```python
from build123d import *

# Parameters (mm, degrees)
SKETCH_1_W                = 50.28
SKETCH_1_H                = 34.2
SKETCH_1_W_2              = 30.28
SKETCH_1_H_2              = 14.2
EXTRUDE_1_DEPTH           = 12.25
SKETCH_4_W                = 13
SKETCH_4_H                = 13.91
EXTRUDE_1_2_DEPTH         = 74.82
SKETCH_5_W                = 13.91
SKETCH_5_H                = 16.23
EXTRUDE_2_DEPTH           = 16
SKETCH_7_R                = 25.25
SKETCH_7_R_2              = 15.25
EXTRUDE_2_2_DEPTH         = 16.23
SKETCH_15_R               = 1.91
CUT_EXTRUDE_6_DEPTH       = 97.964478439
SKETCH_18_W               = 49.344544624
SKETCH_18_H               = 6.125
CUT_EXTRUDE_8_DEPTH       = 101.789238284
SKETCH_19_W               = 34.2
SKETCH_19_H               = 6.125
CUT_EXTRUDE_9_DEPTH       = 10
SKETCH_21_R               = 1.91
CUT_EXTRUDE_10_DEPTH      = 10
SKETCH_20_R               = 1.91
CUT_EXTRUDE_11_DEPTH      = 10
FILLET_START              = -7.1
FILLET_1_DEPTH            = 14.2
FILLET_2_DEPTH            = 14.2
SKETCH_29_W               = 13.91
SKETCH_29_H               = 74.82
EXTRUDE_5_DEPTH           = 10
SKETCH_30_W               = 10
SKETCH_30_H               = 58.59
CUT_EXTRUDE_13_DEPTH      = 97.964478439
SKETCH_32_W               = 34.2
SKETCH_32_H               = 5.745736365
EXTRUDE_6_DEPTH           = 10
CUT_EXTRUDE_16_DEPTH      = 50
CUT_EXTRUDE_16_DEPTH_BACK = 50
SKETCH_38_W               = 116.985630298
SKETCH_38_H               = 80.538350638
SKETCH_41_W               = 13.91
SKETCH_41_H               = 5.745736365
EXTRUDE_7_DEPTH           = 3
SKETCH_42_W               = 13
SKETCH_42_H               = 13.91
EXTRUDE_8_DEPTH           = 74.82
SKETCH_43_W               = 13.91
SKETCH_43_H               = 16.23
EXTRUDE_9_DEPTH           = 15.22
SKETCH_44_R               = 1.91
CUT_EXTRUDE_17_DEPTH      = 15.22
SKETCH_46_R               = 25.25
SKETCH_46_R_2             = 15.25
EXTRUDE_6_2_DEPTH         = 16.23
EXTRUDE_10_DEPTH          = 7.22
EXTRUDE_10_DEPTH_BACK     = 10
SKETCH_47_W               = 13.91
SKETCH_47_H               = 16.23
SKETCH_50_W               = 3.056753925
SKETCH_50_H               = 16.23
CUT_EXTRUDE_18_DEPTH      = 96.578211037
SKETCH_51_R               = 1.91
CUT_EXTRUDE_19_DEPTH      = 95.015226304
SKETCH_52_W               = 92.841945613
SKETCH_52_H               = 30
CUT_EXTRUDE_20_DEPTH      = 84.840694713
CUT_EXTRUDE_22_DEPTH      = 50
CUT_EXTRUDE_22_DEPTH_BACK = 50
SKETCH_53_W               = 63.541345486
SKETCH_53_H               = 14.170740414
SKETCH_54_W               = 10
SKETCH_54_H               = 10.145
CUT_EXTRUDE_23_DEPTH      = 50
SKETCH_55_W               = 13
SKETCH_55_H               = 13.91
EXTRUDE_11_DEPTH          = 10
SKETCH_57_W               = 15
SKETCH_57_H               = 34.2
EXTRUDE_12_DEPTH          = 10
SKETCH_58_W               = 34.2
SKETCH_58_H               = 10
EXTRUDE_13_DEPTH          = 27.85
SKETCH_60_W               = 34.2
SKETCH_60_H               = 10
EXTRUDE_14_DEPTH          = 50.28
SKETCH_62_W               = 30.28
SKETCH_62_H               = 14.2
CUT_EXTRUDE_24_DEPTH      = 50.28
SKETCH_64_R               = 1.91
CUT_EXTRUDE_25_DEPTH      = 10
FILLET_3_R                = 30


with BuildPart() as part:
    # 草圖1 → Extrude 1 (new body)
    with BuildSketch(Plane(origin=(0, 0, 0), x_dir=(1, 0, 0), z_dir=(0, 1, 0))):
        Rectangle(SKETCH_1_W, SKETCH_1_H)
        Rectangle(SKETCH_1_W_2, SKETCH_1_H_2, mode=Mode.SUBTRACT)
    extrude(amount=EXTRUDE_1_DEPTH)

    # 草圖4 → Extrude 1 2 (add)
    with BuildSketch(Plane.XZ):
        with Locations((18.64, 0)):
            Rectangle(SKETCH_4_W, SKETCH_4_H)
    extrude(amount=EXTRUDE_1_2_DEPTH)

    # 草圖5 → Extrude 2 (add)
    with BuildSketch(Plane.ZY.offset(-12.14)):
        with Locations((0, -66.705)):
            Rectangle(SKETCH_5_W, SKETCH_5_H)
    extrude(amount=EXTRUDE_2_DEPTH)

    # 草圖7 → Extrude 2 2 (add)
    with BuildSketch(Plane(origin=(3.626674765, -74.82, 0), x_dir=(1, 0, 0), z_dir=(0, -1, 0))):
        with Locations((-30.978154344, 0)):
            Circle(SKETCH_7_R)
        with Locations((-30.978154344, 0)):
            Circle(SKETCH_7_R_2, mode=Mode.SUBTRACT)
    extrude(amount=-EXTRUDE_2_2_DEPTH)

    # 草圖15 → 除料-伸長6 (cut, through all)
    with BuildSketch(Plane(origin=(0, 0, -6.955), x_dir=(-1, 0, 0), z_dir=(0, 0, -1))):
        with Locations((-4.530883248, -66.705)):
            Circle(SKETCH_15_R)
    extrude(amount=-CUT_EXTRUDE_6_DEPTH, mode=Mode.SUBTRACT)

    # 草圖18 → 除料-伸長8 (cut, through all)
    with BuildSketch(Plane(origin=(0, 0, -17.1), x_dir=(-1, 0, 0), z_dir=(0, 0, -1))):
        with Locations((0.467727688, 9.1875)):
            Rectangle(SKETCH_18_W, SKETCH_18_H)
    extrude(amount=-CUT_EXTRUDE_8_DEPTH, mode=Mode.SUBTRACT)

    # 草圖19 → 除料-伸長9 (cut)
    with BuildSketch(Plane.ZY.offset(-24.204544624)):
        with Locations((0, 9.1875)):
            Rectangle(SKETCH_19_W, SKETCH_19_H)
    extrude(amount=-CUT_EXTRUDE_9_DEPTH, mode=Mode.SUBTRACT)

    # 草圖21 → 除料-伸長10 (cut)
    with BuildSketch(Plane(origin=(0, 6.125, 0), x_dir=(1, 0, 0), z_dir=(0, 1, 0))):
        with Locations(Location((17.69, 0, 0), (0, 0, 270))):
            Circle(SKETCH_21_R)
    extrude(amount=-CUT_EXTRUDE_10_DEPTH, mode=Mode.SUBTRACT)

    # 草圖20 → 除料-伸長11 (cut)
    with BuildSketch(Plane(origin=(0, 6.125, 0), x_dir=(1, 0, 0), z_dir=(0, 1, 0))):
        with Locations(Location((-17.395, 0, 0), (0, 0, 270))):
            Circle(SKETCH_20_R)
    extrude(amount=-CUT_EXTRUDE_11_DEPTH, mode=Mode.SUBTRACT)

    # 圓角1: read off the stored shape, not the designer's step
    # 圓角1 outline → 圓角1 (cut)
    with BuildSketch(Plane.XY.offset(FILLET_START)):
        with BuildLine():
            add(Edge.make_bspline(
                [(-15.14, 0), (-21.974170252, 5.199829476), (-25.14, 5.745736365)],
                knots=[0, 0, 0, 0.664102345, 0.664102345, 0.664102345], degree=2, weights=[1, 2.223777218, 1.822127795]))
            Line((-15.14, 0), (-15.14, 6.125))
            Line((-15.14, 6.125), (-25.14, 6.125))
            Line((-25.14, 6.125), (-25.14, 5.745736365))
        make_face()
    extrude(amount=FILLET_1_DEPTH, mode=Mode.SUBTRACT)

    # 圓角2: read off the stored shape, not the designer's step
    # 圓角2 outline → 圓角2 (cut)
    with BuildSketch(Plane.XY.offset(FILLET_START)):
        with BuildLine():
            Line((15.14, 6.125), (15.14, 0))
            add(Edge.make_bspline(
                [(15.14, 0), (21.974170252, 5.199829476), (25.14, 5.745736365)],
                knots=[0, 0, 0, 0.664102345, 0.664102345, 0.664102345], degree=2, weights=[1, 2.223777218, 1.822127795]))
            Line((25.14, 5.745736365), (25.14, 6.125))
            Line((25.14, 6.125), (15.14, 6.125))
        make_face()
    extrude(amount=FILLET_2_DEPTH, mode=Mode.SUBTRACT)

    # 草圖29 → 填料-伸長5 (add)
    with BuildSketch(Plane(origin=(25.14, 0, 0), x_dir=(0, 0, -1), z_dir=(1, 0, 0))):
        with Locations((0, -37.41)):
            Rectangle(SKETCH_29_W, SKETCH_29_H)
    extrude(amount=EXTRUDE_5_DEPTH)

    # 草圖30 → 除料-伸長13 (cut, through all)
    with BuildSketch(Plane.XY.offset(6.955)):
        with Locations((17.14, -29.295)):
            Rectangle(SKETCH_30_W, SKETCH_30_H)
    extrude(amount=-CUT_EXTRUDE_13_DEPTH, mode=Mode.SUBTRACT)

    # 草圖32 → Extrude 6 (add)
    with BuildSketch(Plane(origin=(25.14, 0, 0), x_dir=(0, 0, -1), z_dir=(1, 0, 0))):
        with Locations((0, 2.872868182)):
            Rectangle(SKETCH_32_W, SKETCH_32_H)
    extrude(amount=EXTRUDE_6_DEPTH)

    # 草圖38 → 除料-伸長16 (cut, two sides: drawn at the far end of the back side and taken through both)
    with BuildSketch(Plane(origin=(0, 0, -6.955), x_dir=(-1, 0, 0), z_dir=(0, 0, -1)).offset(-CUT_EXTRUDE_16_DEPTH_BACK)):
        with Locations((7.268869252, -40.269175319)):
            Rectangle(SKETCH_38_W, SKETCH_38_H)
    extrude(amount=CUT_EXTRUDE_16_DEPTH + CUT_EXTRUDE_16_DEPTH_BACK, mode=Mode.SUBTRACT)

    # 草圖41 → 填料-伸長7 (add)
    with BuildSketch(Plane(origin=(35.14, 0, 0), x_dir=(0, 0, -1), z_dir=(1, 0, 0))):
        with Locations((0, 2.872868182)):
            Rectangle(SKETCH_41_W, SKETCH_41_H)
    extrude(amount=EXTRUDE_7_DEPTH)

    # 草圖42 → 填料-伸長8 (add)
    with BuildSketch(Plane(origin=(0, 0, 0), x_dir=(-1, 0, 0), z_dir=(0, -1, 0))):
        with Locations((-31.64, 0)):
            Rectangle(SKETCH_42_W, SKETCH_42_H)
    extrude(amount=EXTRUDE_8_DEPTH)

    # 草圖43 → 填料-伸長9 (add)
    with BuildSketch(Plane.ZY.offset(-25.14)):
        with Locations((0, -66.705)):
            Rectangle(SKETCH_43_W, SKETCH_43_H)
    extrude(amount=EXTRUDE_9_DEPTH)

    # 草圖44 → 除料-伸長17 (cut)
    with BuildSketch(Plane(origin=(0, 0, -6.955), x_dir=(-1, 0, 0), z_dir=(0, 0, -1))):
        with Locations(Location((-17.524895264, -66.705, 0), (0, 0, 90))):
            Circle(SKETCH_44_R)
    extrude(amount=-CUT_EXTRUDE_17_DEPTH, mode=Mode.SUBTRACT)

    # 草圖46 → Extrude 6 2 (add)
    with BuildSketch(Plane(origin=(0, -58.59, 0), x_dir=(1, 0, 0), z_dir=(0, 1, 0))):
        with Locations((-14.35, 0)):
            Circle(SKETCH_46_R)
        with Locations((-14.35, 0)):
            Circle(SKETCH_46_R_2, mode=Mode.SUBTRACT)
    extrude(amount=-EXTRUDE_6_2_DEPTH)

    # 草圖47 → 填料-伸長10 (add, two sides: drawn at the far end of the back side and taken through both)
    with BuildSketch(Plane(origin=(-40, 0, 0), x_dir=(0, 0, -1), z_dir=(1, 0, 0)).offset(-EXTRUDE_10_DEPTH_BACK)):
        with Locations((0, -66.705)):
            Rectangle(SKETCH_47_W, SKETCH_47_H)
    extrude(amount=EXTRUDE_10_DEPTH + EXTRUDE_10_DEPTH_BACK)

    # 草圖50 → 除料-伸長18 (cut, through all)
    with BuildSketch(Plane(origin=(0, 0, -6.955), x_dir=(-1, 0, 0), z_dir=(0, 0, -1))):
        with Locations((48.471623038, -66.705)):
            Rectangle(SKETCH_50_W, SKETCH_50_H)
    extrude(amount=-CUT_EXTRUDE_18_DEPTH, mode=Mode.SUBTRACT)

    # 草圖51 → 除料-伸長19 (cut, through all)
    with BuildSketch(Plane(origin=(0, 0, -6.955), x_dir=(-1, 0, 0), z_dir=(0, 0, -1))):
        with Locations((42.786508152, -66.705)):
            Circle(SKETCH_51_R)
    extrude(amount=-CUT_EXTRUDE_19_DEPTH, mode=Mode.SUBTRACT)

    # 草圖52 → 除料-伸長20 (cut, through all)
    with BuildSketch(Plane(origin=(0, -58.59, 0), x_dir=(1, 0, 0), z_dir=(0, 1, 0))):
        with Locations((-21.280972807, 15)):
            Rectangle(SKETCH_52_W, SKETCH_52_H)
    extrude(amount=-CUT_EXTRUDE_20_DEPTH, mode=Mode.SUBTRACT)

    # 草圖53 → 除料-伸長22 (cut, two sides: drawn at the far end of the back side and taken through both)
    with BuildSketch(Plane(origin=(0, 0, -6.955), x_dir=(-1, 0, 0), z_dir=(0, 0, -1)).offset(-CUT_EXTRUDE_22_DEPTH_BACK)):
        with Locations((6.630672743, -0.960370207)):
            Rectangle(SKETCH_53_W, SKETCH_53_H)
    extrude(amount=CUT_EXTRUDE_22_DEPTH + CUT_EXTRUDE_22_DEPTH_BACK, mode=Mode.SUBTRACT)

    # 草圖54 → 除料-伸長23 (cut)
    with BuildSketch(Plane(origin=(0, 5.745736365, 0), x_dir=(1, 0, 0), z_dir=(0, 1, 0))):
        with Locations((30.14, -12.0275)):
            Rectangle(SKETCH_54_W, SKETCH_54_H)
        with Locations((30.14, 12.0275)):
            Rectangle(SKETCH_54_W, SKETCH_54_H)
    extrude(amount=-CUT_EXTRUDE_23_DEPTH, mode=Mode.SUBTRACT)

    # 草圖55 → 填料-伸長11 (add)
    with BuildSketch(Plane(origin=(0, 5.745736365, 0), x_dir=(1, 0, 0), z_dir=(0, 1, 0))):
        with Locations((31.64, 0)):
            Rectangle(SKETCH_55_W, SKETCH_55_H)
    extrude(amount=EXTRUDE_11_DEPTH)

    # 草圖57 → 填料-伸長12 (add)
    with BuildSketch(Plane(origin=(0, 15.745736365, 0), x_dir=(1, 0, 0), z_dir=(0, 1, 0))):
        with Locations((31.64, 0)):
            Rectangle(SKETCH_57_W, SKETCH_57_H)
    extrude(amount=EXTRUDE_12_DEPTH)

    # 草圖58 → 填料-伸長13 (add)
    with BuildSketch(Plane.ZY.offset(-24.14)):
        with Locations((0, 20.745736365)):
            Rectangle(SKETCH_58_W, SKETCH_58_H)
    extrude(amount=EXTRUDE_13_DEPTH)

    # 草圖60 → 填料-伸長14 (add)
    with BuildSketch(Plane.ZY.offset(3.71)):
        with Locations((0, 20.745736365)):
            Rectangle(SKETCH_60_W, SKETCH_60_H)
    extrude(amount=EXTRUDE_14_DEPTH)

    # 草圖62 → 除料-伸長24 (cut)
    with BuildSketch(Plane(origin=(0, 25.745736365, 0), x_dir=(1, 0, 0), z_dir=(0, 1, 0))):
        with Locations((-28.85, 0)):
            Rectangle(SKETCH_62_W, SKETCH_62_H)
    extrude(amount=-CUT_EXTRUDE_24_DEPTH, mode=Mode.SUBTRACT)

    # 草圖64 → 除料-伸長25 (cut)
    with BuildSketch(Plane(origin=(0, 25.745736365, 0), x_dir=(1, 0, 0), z_dir=(0, 1, 0))):
        with Locations(Location((-8.71, 0, 0), (0, 0, 270))):
            Circle(SKETCH_64_R)
        with Locations(Location((-48.99, 0, 0), (0, 0, 270))):
            Circle(SKETCH_64_R)
    extrude(amount=-CUT_EXTRUDE_25_DEPTH, mode=Mode.SUBTRACT)

    # 圓角3
    # the kernel refuses this fillet: 30 mm, written as the material it takes off along each edge
    with BuildSketch(Plane(origin=(-43.99, 25.745736365, 7.1), x_dir=(-1, 0, 0), z_dir=(0, 0, -1)), Plane(origin=(-13.71, 25.745736365, -7.1), x_dir=(1, 0, 0), z_dir=(0, 0, 1))) as fillet_3_piece_1:
        with BuildLine():
            CenterArc((22.360679775, -30), FILLET_3_R, 90, 48.189685104)
            Line((0, -10), (0, 0))
            Line((0, 0), (22.360679775, 0))
        make_face()
    extrude(amount=14.2, mode=Mode.SUBTRACT)


solid = part.part
```
Source: CAD feature listing. Evaluate the final solid. Frame: model axes, mm. A direction names the side the tool comes from. Round coordinates to 2 decimals unless told otherwise and drop trailing zeros. Write each loop counter-clockwise with the first axis right and the second up, starting at its lowest first coordinate (ties: lowest second). Pieces come first, ordered by that corner, then holes. Notation, with made-up numbers: M 9.25,2 L 17.25,2 A16 ccw 17.25,29 Z; hole C 37,82 d10. An arc over 180 degrees is marked long. Answer as a JSON object with one key per item and string values. Group by question number.
(1) Mould query, pull axis X, two halves, no side actions, for faces 1 (the cylindrical face through (-47.575, 19.144, 1.677)), 2 (the flat face through (-46.943, -67, 3)), 3 (the flat face through (13, -67, 0)). Classes: +X half, -X half, draft (parallel to the pull), parting line (faces both ways), or undercut.
(2) Section query D-D on z = -10.5. Output: boundary loops of the cut face in (x, y), then the cut area to 3 significant figures.
(3) Ray query, line 1 (Y direction, x = -31, z = 17); line 2 (X direction, y = -50, z = 6.5); line 3 (X direction, y = 17.1, z = 0). Return the intervals inside material, ascending. Write a range as [from, to].
(4) Section query B-B on x = -19. Output: boundary loops of the cut face in (y, z), then the cut area to 3 significant figures.
(5) First-contact query: pin 1 (7 mm diameter, centred on y = -36, z = -2, fed in from +X); pin 2 (10 mm diameter, centred on x = 24.5, y = 11, fed in from +Z); pin 3 (5.5 mm diameter, centred on y = -69.5, z = 4, fed in from -X); pin 4 (1 mm diameter, centred on x = -8.5, z = -0.5, fed in from -Y). Flat tips, straight axial feed; report the tip coordinate or a pass-through.
(6) Reachability of faces 4 (the cylindrical face through (-14.807, -66.591, 25.246)), 5 (the flat face through (-11, -58.59, 16)), 6 (the flat face through (30, -40, 6.955)), 7 (the flat face through (-7, 21, 17.1)) from +Z, -Z, +X, -X, +Y, -Y: full face, straight path, thin tool, end or side. Return the list, or none.
(7) Section query C-C on x = 32. Output: boundary loops of the cut face in (y, z) (3 decimals).
(8) Section query A-A on x = 13.5. Output: boundary loops of the cut face in (y, z) (3 decimals).
Computed values:
{
 "1": {"face 1": "undercut", "face 2": "-X half", "face 3": "draft"},
 "2": {"outline": "M -53.99,15.75 L 39.14,15.75 L 39.14,25.75 L -53.99,25.75 Z", "area": "931 mm^2"},
 "3": {"line 1": "[-74.82, -58.59], [15.75, 25.75]", "line 2": "[25.14, 38.14]", "line 3": "[-53.99, -50.9], [-47.08, -45.28], [-12.42, -10.62], [-6.8, 39.14]"},
 "4": {"outline": "M -74.82,14.52 L -58.59,14.52 L -58.59,24.82 L -74.82,24.82 Z; M 15.75,-17.1 L 25.75,-17.1 L 25.75,-7.1 L 15.75,-7.1 Z; M 15.75,7.1 L 25.75,7.1 L 25.75,17.1 L 15.75,17.1 Z", "area": "367 mm^2"},
 "5": {"pin 1": "x = 38.14", "pin 2": "z = 17.1", "pin 3": "x = -46.94", "pin 4": "through"},
 "6": {"face 4": "+Z, -Y", "face 5": "+Z, -Z, -X", "face 6": "+Z, +X, -Y", "face 7": "+Z, +X, -X, +Y"},
 "7": {"outline": "M -74.82,-6.955 L 15.746,-6.955 L 15.746,-17.1 L 25.746,-17.1 L 25.746,17.1 L 15.746,17.1 L 15.746,6.955 L -74.82,6.955 Z"},
 "8": {"outline": "M -74.82,0 L -58.59,0 L -58.59,6.955 L -74.82,6.955 Z; M 15.746,-17.1 L 25.746,-17.1 L 25.746,17.1 L 15.746,17.1 Z"}
}
